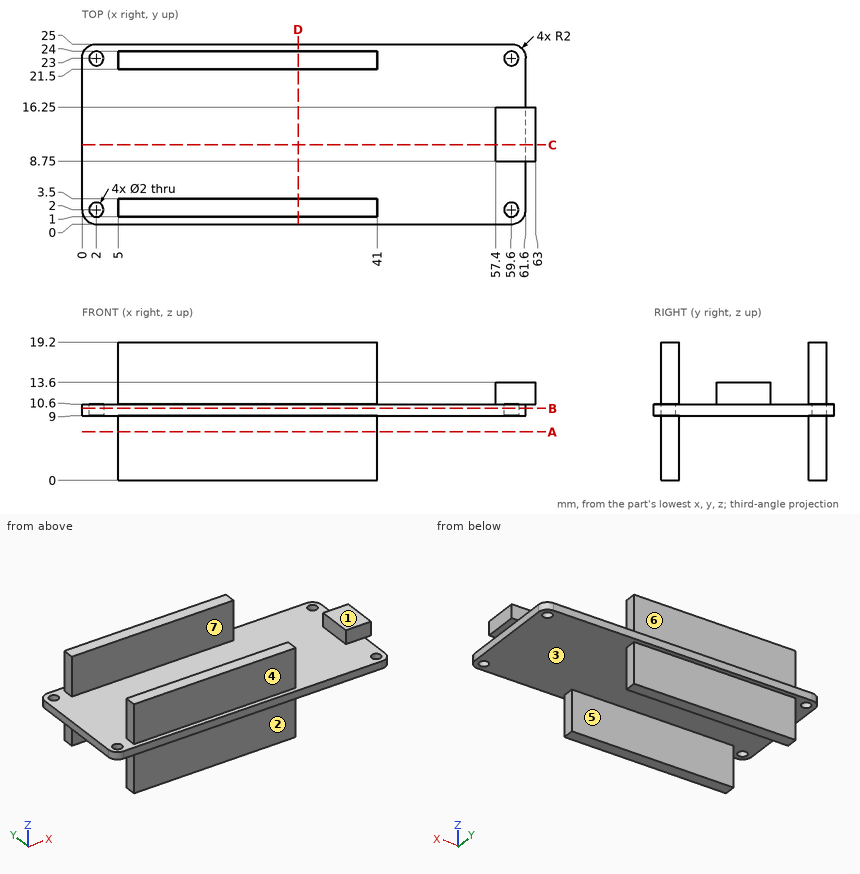
Here's the drawing with two shaded views (mm, measured from the low corner). I have some questions. A direction names the side the tool comes from. Coordinates: 2 decimals unless noted, no trailing zeros. Loops run counter-clockwise (first coordinate to the right, second up) from the corner with the lowest first, then second, coordinate; pieces in that order, holes last. Notation, with made-up numbers: (2, 77) -> (60, 77) arc R6 ccw to (60, 84) -> close; hole circle Ø1 at (-27, 74.25). An arc over 180 degrees is marked (long way). Use one line per item in the form item = value. Start each with the question number.
(1) If we section it at D-D (x = 30): Please give me the cut outline in (y, z).
(2) On a 3-axis mill with a long thin cutter (end or side, diameter ignored), from which of +Z, -Z, +X, -X, +Y, -Y can I reach the whole of each face in a straight line? I mean the marked faces 4, 5, 6 and 7. Say none if no direction works.
(3) Please list where these lines run through material, in increasing order: line 1 along Y through (x, z) = (2, 9.65); line 2 along Y through (x, z) = (10, 15.25); line 3 along Z through (x, y) = (19, 17).
(4) If we section it at C-C (y = 11): Please give me the cut outline in (x, z), then the cut area to 3 significant figures.
(5) We'd pull the mould along Y, two halves only. Please class the marked faces 1, 2 and 3: pulls with the +Y half, pulls with the -Y half, needs draft (parallel to the pull), parting line crosses it, or undercut.
(6) If we section it at B-B (z = 10): Please give me the cut outline in (x, y), then the cut area to 3 significant figures.
(7) Will these pins go through, and if not, where does the flat tip stop? pin 1 (1.5 mm diameter, centred on x = 59.5, z = 12.5, fed in from +Y); pin 2 (2.5 mm diameter, centred on x = 19.5, z = 3.5, fed in from +Y); pin 3 (0.8 mm diameter, centred on y = 23, z = 13.5, fed in from +X).
(8) If we section it at A-A (z = 6.75): Please give me the cut outline in (x, y).
Verdict:
q1.outline = (0, 9) -> (1, 9) -> (1, 0) -> (3.5, 0) -> (3.5, 9) -> (21.5, 9) -> (21.5, 0) -> (24, 0) -> (24, 9) -> (25, 9) -> (25, 10.6) -> (24, 10.6) -> (24, 19.2) -> (21.5, 19.2) -> (21.5, 10.6) -> (3.5, 10.6) -> (3.5, 19.2) -> (1, 19.2) -> (1, 10.6) -> (0, 10.6) -> close
q2.face_4 = +Z, +X, -X, -Y
q2.face_5 = -Z, +X, -X
q2.face_6 = +Z, +X, -X, +Y
q2.face_7 = +Z, +X, -X
q3.line_1 = 0 to 1, 3 to 22, 24 to 25
q3.line_2 = 1 to 3.5, 21.5 to 24
q3.line_3 = 9 to 10.6
q4.outline = (0, 9) -> (61.6, 9) -> (61.6, 10.6) -> (63, 10.6) -> (63, 13.6) -> (57.4, 13.6) -> (57.4, 10.6) -> (0, 10.6) -> close
q4.area = 115 mm²
q5.face_1 = needs draft
q5.face_2 = pulls with the -Y half
q5.face_3 = undercut
q6.outline = (0, 2) arc R2 ccw to (2, 0) -> (59.6, 0) arc R2 ccw to (61.6, 2) -> (61.6, 23) arc R2 ccw to (59.6, 25) -> (2, 25) arc R2 ccw to (0, 23) -> close; hole circle Ø2 at (2, 2); hole circle Ø2 at (2, 23); hole circle Ø2 at (59.6, 2); hole circle Ø2 at (59.6, 23)
q6.area = 1,520 mm²
q7.pin_1 = 16.25
q7.pin_2 = 24
q7.pin_3 = 41
q8.outline = (5, 1) -> (41, 1) -> (41, 3.5) -> (5, 3.5) -> close; (5, 21.5) -> (41, 21.5) -> (41, 24) -> (5, 24) -> close
